Geometry: see drawing. Coordinates: mm, zero at the bounding-box minimum. A direction names the side the tool comes from. Coordinates: 2 decimals unless noted, no trailing zeros. Write each loop counter-clockwise with the first axis right and the second up, starting at its lowest first coordinate (ties: lowest second). Pieces come first, ordered by that corner, then holes.
1) Set-up query: the marked faces 4, 5 and 6. Return all of +Z, -Z, +X, -X, +Y, -Y with unobstructed straight access to the full face (end or side cutting, diameter ignored); none if empty.
2) Draft query along Z for the marked faces 1, 2 and 3. Return one class per face: pulls with the +Z half, pulls with the -Z half, needs draft (parallel to the pull), parting line crosses it, or undercut.
3) Line query: L1, parallel to Y at x = 1.85, z = 13.5; L2, parallel to Y at x = 7.75, z = 13.5; L3, parallel to Z at x = 20.5, y = 40. Output: solid intervals per line, ascending.
4) Pin query (flat end, axial travel): pin 1 Ø1.2 at (x, z) = (15.5, 24.5) entering from -Y; pin 2 Ø1.5 at (y, z) = (22.5, 12) entering from +X; pin 3 Ø0.5 at (x, z) = (20.5, 1.5) entering from +Y; pin 4 Ø8 at (y, z) = (7, 23) entering from -X. Return the tip coordinate at first contact, or that it passes through.
5) Section query B-B (z = 13.5). Output: boundary loops of the cut face in (x, y).
6) Section query C-C (x = 4.5). Output: boundary loops of the cut face in (y, z), then the cut area to 3 significant figures.
7) Section query A-A (x = 11). Output: boundary loops of the cut face in (y, z), then the cut area to 3 significant figures.
8) Section query D-D (z = 2.5). Output: boundary loops of the cut face in (x, y), then the cut area to 3 significant figures.
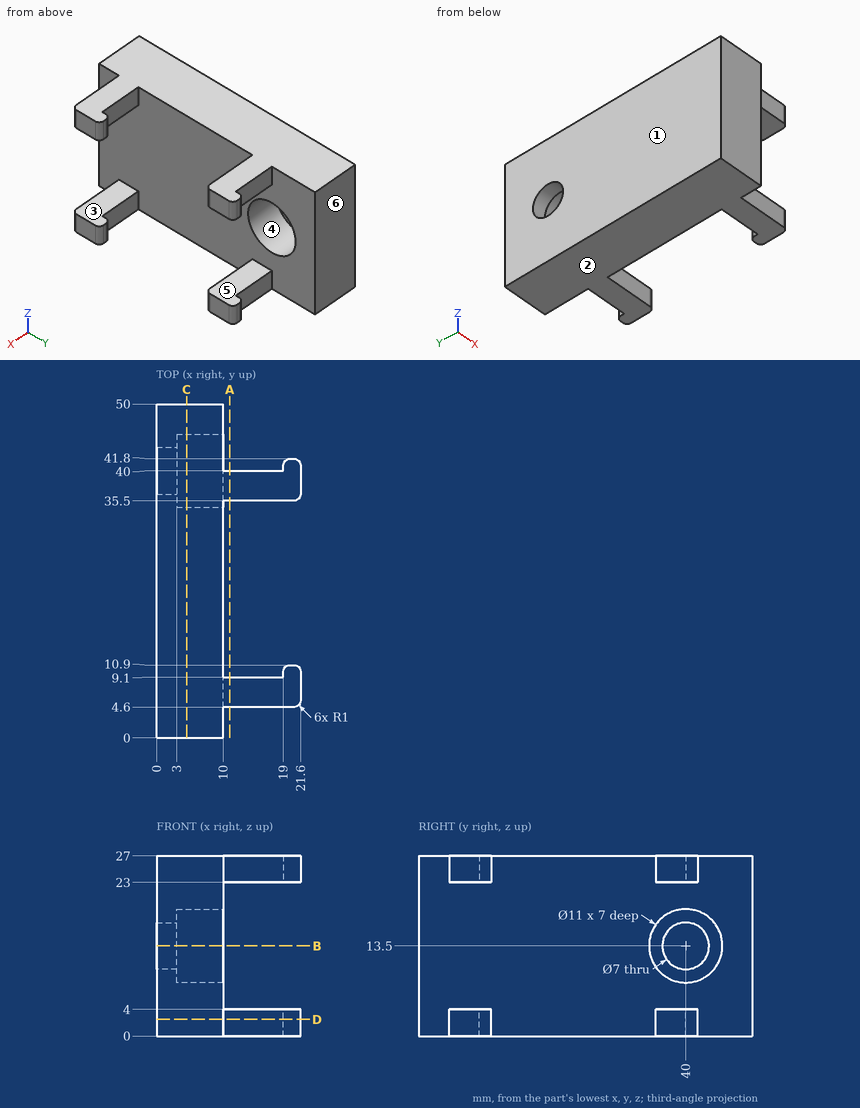
Answer:
1. face 4: +X
1. face 5: +X, +Y, -Y
1. face 6: +Z, -Z, +X, -X, +Y
2. face 1: needs draft
2. face 2: pulls with the -Z half
2. face 3: undercut
3. L1: y = 0 to 36.5, 43.5 to 50
3. L2: y = 0 to 34.5, 45.5 to 50
3. L3: z = 0 to 4, 23 to 27
4. pin 1: stops at y = 4.6
4. pin 2: stops at x = 10
4. pin 3: stops at y = 41.8
4. pin 4: stops at x = 0
5. outline: (0, 0) - (10, 0) - (10, 34.5) - (3, 34.5) - (3, 36.5) - (0, 36.5) - close; (0, 43.5) - (3, 43.5) - (3, 45.5) - (10, 45.5) - (10, 50) - (0, 50) - close
6. outline: (0, 0) - (50, 0) - (50, 27) - (0, 27) - close; hole circle Ø11 at (40, 13.5)
6. area: 1,250 mm2
7. outline: (4.6, 0) - (9.1, 0) - (9.1, 4) - (4.6, 4) - close; (4.6, 23) - (9.1, 23) - (9.1, 27) - (4.6, 27) - close; (35.5, 0) - (40, 0) - (40, 4) - (35.5, 4) - close; (35.5, 23) - (40, 23) - (40, 27) - (35.5, 27) - close
7. area: 72.0 mm2
8. outline: (0, 0) - (10, 0) - (10, 4.6) - (20.6, 4.6) arc R1 ccw to (21.6, 5.6) - (21.6, 9.9) arc R1 ccw to (20.6, 10.9) - (20, 10.9) arc R1 ccw to (19, 9.9) - (19, 9.1) - (10, 9.1) - (10, 35.5) - (20.6, 35.5) arc R1 ccw to (21.6, 36.5) - (21.6, 40.8) arc R1 ccw to (20.6, 41.8) - (20, 41.8) arc R1 ccw to (19, 40.8) - (19, 40) - (10, 40) - (10, 50) - (0, 50) - close
8. area: 612 mm2
